For this review, take the finished solid that the model builds, in its own axes (mm). A direction names the side the tool comes from. Give positions to 0.01 mm unless a question says otherwise; leave off trailing zeros. Write each loop counter-clockwise with the first axis right and the second up, starting at its lowest first coordinate (ties: lowest second). Pieces come first, ordered by that corner, then holes. Notation, with made-up numbers: (33, 35.25) -> (47, 35.25) arc R16 ccw to (47, 54.25) -> close; hole circle Ø8 at (-6.5, -33). An arc over 180 degrees is marked (long way). Write item = value, one per line.
```python
from build123d import *

# Parameters (mm, degrees)
FILLET_1_R          = 0.2
CUT_EXTRUDE_1_DEPTH = 1.5
SKETCH_3_R          = 1.5
EXTRUDE_1_DEPTH     = 4
CHAMFER_1_SIZE      = 0.5


with BuildPart() as part:
    # 草图1 → 旋转1 (revolve)
    with BuildSketch(Plane.XY):
        with BuildLine():
            Line((0, 0), (0, 2))
            Line((0, 2), (1.3, 2))
            ThreePointArc((1.3, 2), (2.370691821, 1.250626571), (2.75, 0))
            Line((2.75, 0), (0, 0))
        make_face()
    revolve(axis=Axis((0, 0, 0), (0, 1, 0)))

    # 圆角1
    fillet_1_edges = [part.edges().sort_by_distance(p)[0] for p in [
        (-2.75, 0, 0),
    ]]
    fillet(fillet_1_edges, radius=FILLET_1_R)

    # 草图2 → 切除-拉伸1 (cut)
    with BuildSketch(Plane(origin=(0, 2, 0), x_dir=(1, 0, 0), z_dir=(0, 1, 0))):
        Polygon((1.327905619, 0), (0.66395281, 1.15), (-0.66395281, 1.15), (-1.327905619, 0), (-0.66395281, -1.15), (0.66395281, -1.15), align=None)
    extrude(amount=-CUT_EXTRUDE_1_DEPTH, mode=Mode.SUBTRACT)

    # 草图3 → 凸台-拉伸1 (add)
    with BuildSketch(Plane.XZ):
        Circle(SKETCH_3_R)
    extrude(amount=EXTRUDE_1_DEPTH)

    # 倒角1
    chamfer_1_edges = [part.edges().sort_by_distance(p)[0] for p in [
        (-1.5, -4, 0),
    ]]
    chamfer(chamfer_1_edges, length=CHAMFER_1_SIZE)


solid = part.part
```
(1) Take a section at A-A (y = -0.25). Write out the cut boundary in (x, z), plus the area to 3 significant figures.
Answers below:
outline = circle Ø3 at (0, 0)
area = 7.07 mm^2
(2) To check wall thickness, follow probe 1 along Z at (x, y) = (-1.25, 0.75); probe 2 along X at (y, z) = (1, 1); probe 3 along Z at (x, y) = (1, 1). State the ranges of each line that lie inside material, in increasing order.
Answers below:
probe_1 = -2.32 to -0.13, 0.13 to 2.32
probe_2 = -2.32 to -0.75, 0.75 to 2.32
probe_3 = -2.32 to -0.57, 0.57 to 2.32
(3) The part is to be moulded in two halves that separate along Z. For faces 3 (the face through (-1.5, -1.73, 0.07)), 4 (the face through (0, -4, 0)), 5 (the face through (0, 1, -1.15)), say which applies: released by +Z, released by -Z, zero draft, split by the parting line, or undercut.
Answers below:
face_3 = split by the parting line
face_4 = zero draft
face_5 = undercut
(4) For pin 1 (1.5 mm diameter, centred on x = 2, y = -1.5, fed in from -Z); pin 2 (2.5 mm diameter, centred on x = 0, z = -0.5, fed in from +Y); pin 3 (0.7 mm diameter, centred on x = 0.5, y = 1.5, fed in from +Z); pin 4 (2 mm diameter, centred on y = 1, z = -1.5, fed in from +X), all flat-tipped, find the tip position at first contact; note any pin that passes through.
Answers below:
pin_1 = -0.83
pin_2 = 2
pin_3 = 2.4
pin_4 = 2.63
(5) Tool access review of faces 1 (the face through (0, 0, 2)), 2 (the face through (-0.991, 1.26, -0.583)): name each direction out of +Z, -Z, +X, -X, +Y, -Y from which nothing blocks a thin tool from reaching the whole face with its end or side.
Answers below:
face_1 = -Y
face_2 = +Y
